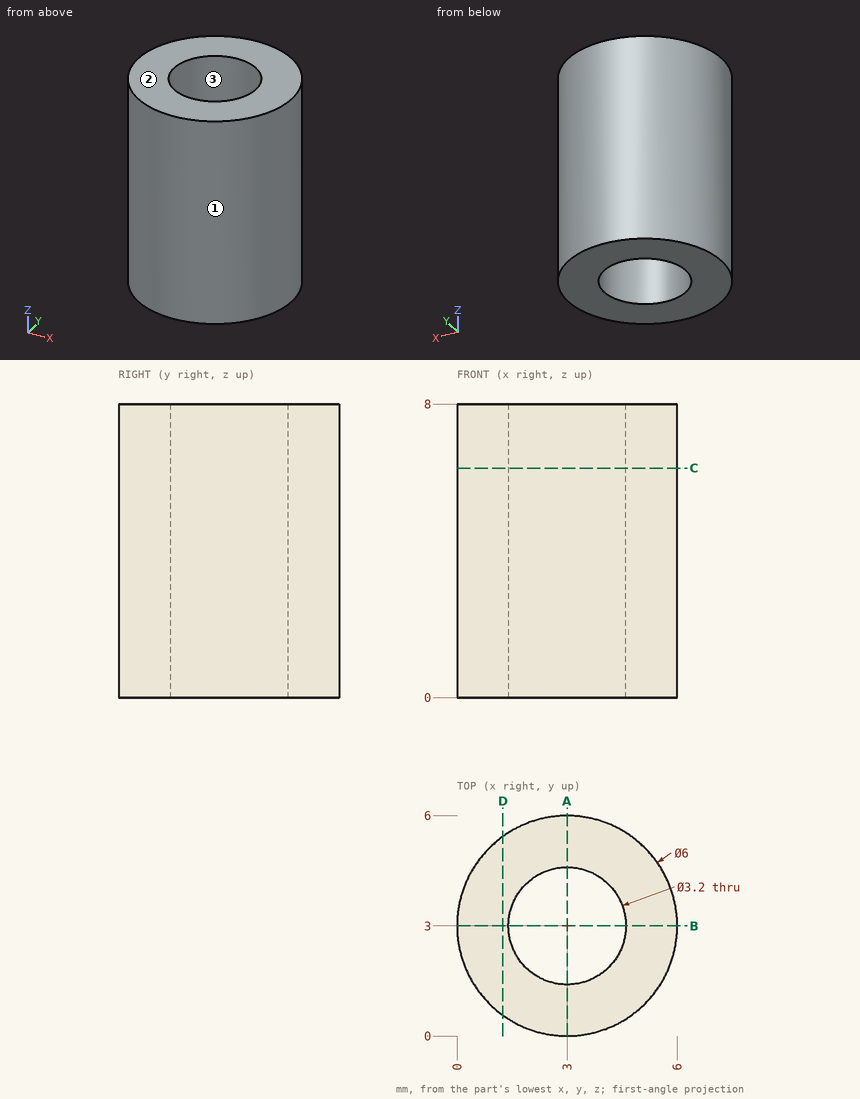
Can you work these out from the drawing? Everything is in mm from the part's minimum corner. Give positions to 0.01 mm unless a question says otherwise; leave off trailing zeros. Loops run counter-clockwise (first coordinate to the right, second up) from the corner with the lowest first, then second, coordinate; pieces in that order, holes last. Notation, with made-up numbers: M -2.5,3 L 19.5,3 A8 cw 19.5,17 Z; hole C 69.25,-6.75 d4. An arc over 180 degrees is marked long. Use CSV: the item, a comma, the result in double quotes. Start each with the question number.
1. Imagine slicing it at C-C, the plane z = 6.25. Write out the boundary of the cut face in (x, y), plus the area to 3 significant figures.
2. Imagine slicing it at A-A, the plane x = 3. Write out the boundary of the cut face in (y, z).
3. For P1, Ø3, axis at x = 3, y = 3, coming from the -Z side; P2, Ø2, axis at x = 5.5, z = 6, coming from the -Y side, each with a flat end and sliding along its axis, tell me the tip position at first contact or that it passes through.
4. If we mould it in two halves opening along Y, with no side actions, what happens to the marked faces 1, 2 and 3? For each: released by +Y, released by -Y, zero draft, split by the parting line, or undercut.
5. Imagine slicing it at D-D, the plane x = 1.25. Write out the boundary of the cut face in (y, z), plus the area to 3 significant figures.
6. If I drill on L1, parallel to Y at x = 3, z = 6; L2, parallel to X at y = 1.9, z = 2; L3, parallel to Y at x = 2.6, z = 2, over which ranges is the centre line in solid material (lowest first)?
Response values:
1,outline,"C 3,3 d6; hole C 3,3 d3.2"
1,area,"20.2 mm^2"
2,outline,"M 0,0 L 1.4,0 L 1.4,8 L 0,8 Z; M 4.6,0 L 6,0 L 6,8 L 4.6,8 Z"
3,P1,"through"
3,P2,"y = 0.4"
4,face 1,"split by the parting line"
4,face 2,"zero draft"
4,face 3,"undercut"
5,outline,"M 0.56,0 L 5.44,0 L 5.44,8 L 0.56,8 Z"
5,area,"39.0 mm^2"
6,L1,"0 to 1.4, 4.6 to 6"
6,L2,"0.21 to 1.84, 4.16 to 5.79"
6,L3,"0.03 to 1.45, 4.55 to 5.97"
